The listing builds one solid part. Answer for the finished solid, in the listing's coordinates (mm). Face numbers are marked on the shaded views. A direction names the side the tool comes from. Coordinates: 2 decimals unless noted, no trailing zeros. Order: outer loops, then holes, each group sorted by start corner. A loop starts at its lowest first (then second) coordinate and runs counter-clockwise, first axis right, second up. Notation, with made-up numbers: (-11.5, 28) -> (24.5, 28) arc R8 ccw to (24.5, 36) -> close; hole circle Ø10 at (34.5, 62.25). An arc over 180 degrees is marked (long way). Answer in a Markdown table with one row per item.
```python
from build123d import *

# Parameters (mm, degrees)
SKETCH_1_W          = 25.5
SKETCH_1_H          = 7.5
EXTRUDE_1_DEPTH     = 3
SKETCH_2_W          = 6.5
SKETCH_2_H          = 7.5
EXTRUDE_2_DEPTH     = 7
EXTRUDE_3_DEPTH     = 3.75
SKETCH_4_R          = 1.75
CUT_EXTRUDE_1_DEPTH = 29.229969862
FILLET_1_R          = 1


with BuildPart() as part:
    # 草图1 → 凸台-拉伸1 (new body)
    with BuildSketch(Plane.XY):
        Rectangle(SKETCH_1_W, SKETCH_1_H)
        with BuildLine():
            Line((-9, 1.75), (-6, 1.75))
            ThreePointArc((-6, 1.75), (-4.25, 0), (-6, -1.75))
            Line((-6, -1.75), (-9, -1.75))
            ThreePointArc((-9, -1.75), (-10.75, 0), (-9, 1.75))
        make_face(mode=Mode.SUBTRACT)
        with BuildLine():
            Line((6, 1.75), (9, 1.75))
            ThreePointArc((9, 1.75), (10.75, 0), (9, -1.75))
            Line((9, -1.75), (6, -1.75))
            ThreePointArc((6, -1.75), (4.25, 0), (6, 1.75))
        make_face(mode=Mode.SUBTRACT)
    extrude(amount=EXTRUDE_1_DEPTH)

    # 草图2 → 凸台-拉伸2 (add)
    with BuildSketch(Plane(origin=(0, 0, 0), x_dir=(-1, 0, 0), z_dir=(0, 0, -1))):
        Rectangle(SKETCH_2_W, SKETCH_2_H)
    extrude(amount=EXTRUDE_2_DEPTH)

    # 草图3 → 凸台-拉伸3 (add, symmetric)
    with BuildSketch(Plane(origin=(0, 0, 0), x_dir=(1, 0, 0), z_dir=(0, 1, 0))):
        with BuildLine():
            Line((-3.75, 14.596873642), (-3.75, 16.910795209))
            ThreePointArc((-3.75, 16.910795209), (-3.372684391, 4.866077927), (7, 11))
            ThreePointArc((7, 11), (6.133922073, 14.372684391), (3.75, 16.910795209))
            Line((3.75, 16.910795209), (3.75, 14.596873642))
            Line((3.75, 14.596873642), (1.75, 14.596873642))
            ThreePointArc((1.75, 14.596873642), (3.391164992, 13.121320344), (4, 11))
            ThreePointArc((4, 11), (-2.121320344, 7.608835008), (-1.75, 14.596873642))
            Line((-1.75, 14.596873642), (-3.75, 14.596873642))
        make_face()
        with BuildLine():
            ThreePointArc((-1.75, 17.777720856), (-2.78395223, 17.422585926), (-3.75, 16.910795209))
            Line((-3.75, 16.910795209), (-3.75, 14.596873642))
            Line((-3.75, 14.596873642), (-1.75, 14.596873642))
            Line((-1.75, 14.596873642), (-1.75, 17.777720856))
        make_face()
        with BuildLine():
            Line((-1.75, 22.596873642), (-3.75, 22.596873642))
            Line((-3.75, 22.596873642), (-3.75, 16.910795209))
            ThreePointArc((-3.75, 16.910795209), (-2.78395223, 17.422585926), (-1.75, 17.777720856))
            Line((-1.75, 17.777720856), (-1.75, 22.596873642))
        make_face()
        with BuildLine():
            Line((1.75, 22.596873642), (1.75, 17.777720856))
            ThreePointArc((1.75, 17.777720856), (2.78395223, 17.422585926), (3.75, 16.910795209))
            Line((3.75, 16.910795209), (3.75, 22.596873642))
            Line((3.75, 22.596873642), (1.75, 22.596873642))
        make_face()
        with BuildLine():
            ThreePointArc((3.75, 16.910795209), (2.78395223, 17.422585926), (1.75, 17.777720856))
            Line((1.75, 17.777720856), (1.75, 14.596873642))
            Line((1.75, 14.596873642), (3.75, 14.596873642))
            Line((3.75, 14.596873642), (3.75, 16.910795209))
        make_face()
    extrude(amount=EXTRUDE_3_DEPTH, both=True)

    # 草图4 → 切除-拉伸1 (cut, through all)
    with BuildSketch(Plane(origin=(3.75, 0, 0), x_dir=(0, 0, -1), z_dir=(1, 0, 0))):
        with Locations((19.753834426, 0)):
            Circle(SKETCH_4_R)
    extrude(amount=-CUT_EXTRUDE_1_DEPTH, mode=Mode.SUBTRACT)

    # 圆角1
    fillet_1_edges = [part.edges().sort_by_distance(p)[0] for p in [
        (2.75, -3.75, -22.596873642),
        (2.75, 3.75, -22.596873642),
        (-2.75, -3.75, -22.596873642),
        (-2.75, 3.75, -22.596873642),
        (-12.75, -3.75, 1.5),
        (12.75, -3.75, 1.5),
        (12.75, 3.75, 1.5),
        (-12.75, 3.75, 1.5),
    ]]
    fillet(fillet_1_edges, radius=FILLET_1_R)


solid = part.part
```
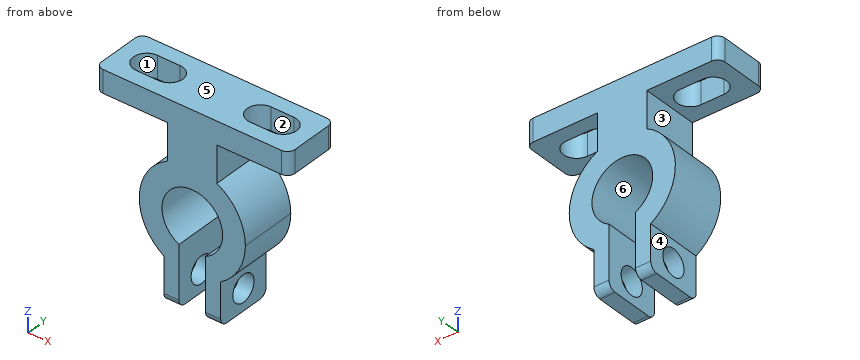
(1) A cutting plane is placed at A-A, the plane x = 7.5. Determine the outline of the cut face in (y, z), then the cut area to 3 significant figures.
Check values:
| item | result |
|---|---|
| outline | (-3.75, 0) -> (-1.75, 0) -> (-1.75, 3) -> (-3.75, 3) -> close; (1.75, 0) -> (3.75, 0) -> (3.75, 3) -> (1.75, 3) -> close |
| area | 12.0 mm² |
(2) A cutting plane is placed at B-B, the plane x = -2.5. Determine the outline of the cut face in (y, z).
Check values:
| item | result |
|---|---|
| outline | (-3.75, -21.6) arc R1 ccw to (-2.75, -22.6) -> (2.75, -22.6) arc R1 ccw to (3.75, -21.6) -> (3.75, -14.12) -> (-3.75, -14.12) -> close; (-3.75, -7.88) -> (3.75, -7.88) -> (3.75, 3) -> (-3.75, 3) -> close; hole circle Ø3.5 at (0, -19.75) |
(3) Find the intervals of material crossed by line 1 along X through (y, z) = (1.75, -10.75); line 2 along Z through (x, y) = (9.5, 3.5); line 3 along X through (y, z) = (2.5, -13.5), in increasing order. Write a range as from..to.
Check values:
| item | result |
|---|---|
| line 1 | -7..-3.99, 3.99..7 |
| line 2 | 0..3 |
| line 3 | -6.54..-3.12, 3.12..6.54 |
(4) A cutting plane is placed at D-D, the plane y = -0.5. Count the separate pieces of the cut face and the enclosed holes in it, then the cut area to 3 significant figures.
Check values:
| item | result |
|---|---|
| separate pieces | 5 |
| enclosed holes | 0 |
| area | 166 mm² |
(5) Which of the six approach directions +Z, -Z, +X, -X, +Y, -Y give full straight-line access (tool end or side, diameter ignored) to the marked faces 1, 2 and 3?
Check values:
| item | result |
|---|---|
| face 1 | +Z, -Z |
| face 2 | +Z |
| face 3 | -X, +Y, -Y |
(6) For a pull along Z with two mould halves and no side action, classify the marked faces 4, 5 and 6 as released by +Z, released by -Z, zero draft, split by the parting line, or undercut.
Check values:
| item | result |
|---|---|
| face 4 | zero draft |
| face 5 | released by +Z |
| face 6 | undercut |
(7) A cutting plane is placed at C-C, the plane z = -15.75. Determine the outline of the cut face in (x, y).
Check values:
| item | result |
|---|---|
| outline | (-5.14, -3.75) -> (-1.75, -3.75) -> (-1.75, 3.75) -> (-5.14, 3.75) -> close; (1.75, -3.75) -> (5.14, -3.75) -> (5.14, 3.75) -> (1.75, 3.75) -> close |
(8) Flat-ended cylindrical pins translate along their axes: pin 1 (1 mm diameter, centred on x = 8, z = -2, fed in from +Y); pin 2 (4 mm diameter, centred on x = -8, y = 0, fed in from -Z); pin 3 (12 mm diameter, centred on x = 4.5, z = -5.5, fed in from -Y); pin 4 (3 mm diameter, centred on y = 0.5, z = -21, fed in from +X). Find the tip coordinate at first contact, or state that the pin passes through.
Check values:
| item | result |
|---|---|
| pin 1 | through |
| pin 2 | z = -14.61 |
| pin 3 | y = -3.75 |
| pin 4 | x = 3.75 |
